```python
from build123d import *

# Parameters (mm, degrees)
F1_DEPTH        = 170
F2_DEPTH        = 20
F4_D            = 7
F6_D            = 6
F6_CSINK_D      = 11.2
F6_CSINK_ANGLE  = 90
F7_DEPTH        = 5
F8_DEPTH        = 5
F9_DEPTH        = 20
F10_D           = 7
F12_D           = 6
F12_CBORE_D     = 8.25
F12_CBORE_DEPTH = 5
F14_D           = 6
F16_D           = 4.2
F16_DEPTH       = 23.4
F16_TIP         = 1.2618073
F17_W           = 180
F17_H           = 14
F17_R           = 3.5
F18_DEPTH       = 4


with BuildPart() as f1:
    # F0 (on Right) → F1 (new body)
    with BuildSketch(Plane.YZ):
        Polygon((0, 170), (0, 0), (20, 0), (20, 400), (0, 400), (0, 185), (5, 185), (5, 170), align=None)
    extrude(amount=F1_DEPTH)

    # F2 (cut): a face of the model
    f2_faces = [f1.faces().sort_by_distance(p)[0] for p in [
        (85, 10, 400),
    ]]
    extrude(f2_faces, amount=-F2_DEPTH, mode=Mode.SUBTRACT)

    # F4 (through all)
    with Locations(Plane(origin=(0, 20, 0), x_dir=(-1, 0, 0), z_dir=(0, 1, 0))):
        with Locations((-165, 197.5), (-165, 157.5), (-5, 197.5), (-5, 157.5), (-112, 197.5), (-112, 157.5), (-58, 157.5), (-58, 197.5)):
            Hole(F4_D / 2)

    # F6 (through all)
    with Locations(Plane(origin=(0, 20, 0), x_dir=(-1, 0, 0), z_dir=(0, 1, 0))):
        with Locations((-151, 177.5), (-118, 177.5), (-85, 177.5), (-52, 177.5), (-19, 177.5)):
            CounterSinkHole(F6_D / 2, F6_CSINK_D / 2, counter_sink_angle=F6_CSINK_ANGLE)

    # F0 (on Right) → F7 (join)
    with BuildSketch(Plane.YZ):
        Polygon((0, 170), (0, 0), (20, 0), (20, 400), (0, 400), (0, 185), (5, 185), (5, 170), align=None)
    extrude(amount=-F7_DEPTH)

    # F8 (add): a face of the model
    f8_faces = [f1.faces().sort_by_distance(p)[0] for p in [
        (170, 10.0747508306, 190.1245847176),
    ]]
    extrude(f8_faces, amount=F8_DEPTH)

    # F9 (cut): a face of the model
    f9_faces = [f1.faces().sort_by_distance(p)[0] for p in [
        (-2.5, 10, 400),
    ]]
    extrude(f9_faces, amount=-F9_DEPTH, mode=Mode.SUBTRACT)

    # F10 (through all)
    with Locations(Plane(origin=(0, 20, 0), x_dir=(-1, 0, 0), z_dir=(0, 1, 0))):
        with Locations((-165, 80), (-165, 40), (-112, 80), (-112, 40), (-58, 40), (-5, 80), (-58, 80), (-5, 40)):
            Hole(F10_D / 2)

    # F12 (through all)
    with Locations(Plane(origin=(0, 20, 0), x_dir=(-1, 0, 0), z_dir=(0, 1, 0))):
        with Locations((-157, 56), (-157, 24), (-121, 56), (-121, 24), (-49, 56), (-49, 24), (-13, 24), (-13, 56)):
            CounterBoreHole(F12_D / 2, F12_CBORE_D / 2, F12_CBORE_DEPTH)

    # F14 (through all)
    with Locations(Plane(origin=(0, 20, 0), x_dir=(-1, 0, 0), z_dir=(0, 1, 0))):
        with Locations((-97, 150), (-97, 110), (-73, 110), (-73, 150)):
            Hole(F14_D / 2)

    # F16
    with Locations(Plane.XY.offset(380)):
        with Locations((15, 10), (50, 10), (85, 10), (120, 10), (155, 10)):
            Hole(F16_D / 2, depth=F16_DEPTH)
            with Locations((0, 0, -(F16_DEPTH + F16_TIP / 2))):  # 118° drill point
                Cone(0, F16_D / 2, F16_TIP, mode=Mode.SUBTRACT)

    # F17 (on face) → F18 (cut)
    with BuildSketch(Plane.XZ):
        with Locations((85, 40)):
            Rectangle(F17_W, F17_H)
        with Locations((5, 40)):
            Circle(F17_R, mode=Mode.SUBTRACT)
        with Locations((58, 40)):
            Circle(F17_R, mode=Mode.SUBTRACT)
        with Locations((112, 40)):
            Circle(F17_R, mode=Mode.SUBTRACT)
        with Locations((165, 40)):
            Circle(F17_R, mode=Mode.SUBTRACT)
    extrude(amount=-F18_DEPTH, mode=Mode.SUBTRACT)


solid = f1.part
```
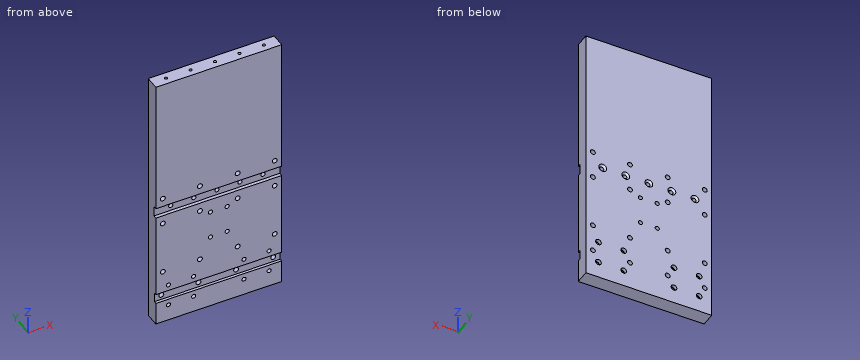
Work out the finished part from the listing and answer in its coordinate system (mm). Give positions to 0.01 mm unless a question says otherwise; leave off trailing zeros. Write each loop counter-clockwise with the first axis right and the second up, starting at its lowest first coordinate (ties: lowest second). Pieces come first, ordered by that corner, then holes. Notation, with made-up numbers: (-25, -30) -> (-6, -30) arc R16 cw to (-6, -7) -> close; hole circle Ø9 at (74.5, 46.5). An arc over 180 degrees is marked (long way). Write each question's results on one line, items separated by ' | '.
1. Straight lines are drawn through the part: L1, parallel to X at y = 10, z = 374.75; L2, parallel to X at y = 13.75, z = 197.5; L3, parallel to Z at x = 165, y = 13.25. For each, find the intervals that lie inside material, in ascending order.
Data:
L1: -5 to 12.9, 17.1 to 47.9, 52.1 to 82.9, 87.1 to 117.9, 122.1 to 152.9, 157.1 to 175 | L2: -5 to 1.5, 8.5 to 54.5, 61.5 to 108.5, 115.5 to 161.5, 168.5 to 175 | L3: 0 to 36.5, 43.5 to 76.5, 83.5 to 154, 161 to 194, 201 to 380
2. Each of these flat-tipped pins is pushed along its axis until it touches: pin 1 Ø4 at (x, z) = (155.5, 23) entering from +Y; pin 2 Ø9.5 at (x, z) = (118, 177.5) entering from +Y; pin 3 Ø3.5 at (x, y) = (15, 10) entering from +Z. Where does it stop, or does it pass through?
Data:
pin 1: y = 15 | pin 2: y = 19.15 | pin 3: z = 356.39
3. Find section A-A on x = 136. Determine the outline of the cut face in (y, z).
Data:
outline: (0, 0) -> (20, 0) -> (20, 380) -> (0, 380) -> (0, 185) -> (5, 185) -> (5, 170) -> (0, 170) -> (0, 47) -> (4, 47) -> (4, 33) -> (0, 33) -> close
